Model file for the job. Use its own axes, mm. A direction names the side the tool comes from. Give positions to 0.01 mm unless a question says otherwise; leave off trailing zeros. Loops run counter-clockwise (first coordinate to the right, second up) from the corner with the lowest first, then second, coordinate; pieces in that order, holes last. Notation, with made-up numbers: (69.5, 3.5) - (82.5, 3.5) arc R35 cw to (82.5, 40.5) - close; hole circle Ø6 at (38, -6). An arc over 180 degrees is marked (long way). Use a Markdown table: item, result.
from build123d import *

# Parameters (mm, degrees)
SKETCH1_W               = 115
SKETCH1_H               = 55
SKETCH1_W_2             = 107
SKETCH1_H_2             = 47
BOSS_EXTRUDE1_DEPTH     = 6
SKETCH2_W               = 5
SKETCH2_H               = 2
BOSS_EXTRUDE2_DEPTH     = 8.5
CUT_EXTRUDE1_DEPTH      = 10
MIRROR2_COPY_1_SKETCH_W = 5
MIRROR2_COPY_1_SKETCH_H = 2
MIRROR2_COPY_1_DEPTH    = 8.5
MIRROR2_COPY_2_DEPTH    = 10
MIRROR3_COPY_1_SKETCH_W = 5
MIRROR3_COPY_1_SKETCH_H = 2
MIRROR3_COPY_1_DEPTH    = 8.5
MIRROR3_COPY_2_DEPTH    = 10
MIRROR3_COPY_3_SKETCH_W = 5
MIRROR3_COPY_3_SKETCH_H = 2
MIRROR3_COPY_3_DEPTH    = 8.5
MIRROR3_COPY_4_DEPTH    = 10
MIRROR3_COPY_5_SKETCH_W = 5
MIRROR3_COPY_5_SKETCH_H = 2
MIRROR3_COPY_5_DEPTH    = 8.5
MIRROR3_COPY_6_DEPTH    = 10


with BuildPart() as part:
    # Sketch1 → Boss-Extrude1 (new body)
    with BuildSketch(Plane.XY):
        Rectangle(SKETCH1_W, SKETCH1_H)
        Rectangle(SKETCH1_W_2, SKETCH1_H_2, mode=Mode.SUBTRACT)
    extrude(amount=BOSS_EXTRUDE1_DEPTH)

    # Sketch2 → Boss-Extrude2 (add)
    with BuildSketch(Plane.XY.offset(6)):
        with Locations((-42.5, 24.5)):
            Rectangle(SKETCH2_W, SKETCH2_H)
    boss_extrude2 = extrude(amount=BOSS_EXTRUDE2_DEPTH)

    # Sketch3 → Cut-Extrude1 (cut)
    with BuildSketch(Plane(origin=(-40, 0, 0), x_dir=(0, 0, -1), z_dir=(1, 0, 0))):
        Polygon((-14.5, 24.5), (-11, 25.5), (-11, 24.633842956), (-6, 24.633842956), (-6, 26.874562864), (-14.5, 26.874562864), align=None)
    cut_extrude1 = extrude(amount=-CUT_EXTRUDE1_DEPTH, mode=Mode.SUBTRACT)

    # Mirror1: Boss-Extrude2, Cut-Extrude1 across plane
    add(boss_extrude2.mirror(Plane.ZX))
    add(cut_extrude1.mirror(Plane.ZX), mode=Mode.SUBTRACT)

    # Mirror2: Boss-Extrude2, Cut-Extrude1 across plane
    add(boss_extrude2.mirror(Plane(origin=(0, 0, 0), x_dir=(0, 0, 1), z_dir=(1, 0, 0))))
    add(cut_extrude1.mirror(Plane(origin=(0, 0, 0), x_dir=(0, 0, 1), z_dir=(1, 0, 0))), mode=Mode.SUBTRACT)

    # Mirror2 copy 1 sketch → Mirror2 copy 1 (add)
    with BuildSketch(Plane(origin=(0, 0, 6), x_dir=(-1, 0, 0), z_dir=(0, 0, 1))):
        with Locations((-42.5, 24.5)):
            Rectangle(MIRROR2_COPY_1_SKETCH_W, MIRROR2_COPY_1_SKETCH_H)
    extrude(amount=MIRROR2_COPY_1_DEPTH)

    # Mirror2 copy 2 sketch → Mirror2 copy 2 (cut)
    with BuildSketch(Plane(origin=(40, 0, 0), x_dir=(0, 0, -1), z_dir=(-1, 0, 0))):
        Polygon((-14.5, 24.5), (-11, 25.5), (-11, 24.633842956), (-6, 24.633842956), (-6, 26.874562864), (-14.5, 26.874562864), align=None)
    extrude(amount=-MIRROR2_COPY_2_DEPTH, mode=Mode.SUBTRACT)

    # Mirror3: Boss-Extrude2, Cut-Extrude1 across plane
    add(boss_extrude2.mirror(Plane.XY.offset(3)))
    add(cut_extrude1.mirror(Plane.XY.offset(3)), mode=Mode.SUBTRACT)

    # Mirror3 copy 1 sketch → Mirror3 copy 1 (add)
    with BuildSketch(Plane(origin=(0, 0, 0), x_dir=(-1, 0, 0), z_dir=(0, 0, -1))):
        with Locations((-42.5, 24.5)):
            Rectangle(MIRROR3_COPY_1_SKETCH_W, MIRROR3_COPY_1_SKETCH_H)
    extrude(amount=MIRROR3_COPY_1_DEPTH)

    # Mirror3 copy 2 sketch → Mirror3 copy 2 (cut)
    with BuildSketch(Plane(origin=(40, 0, 6), x_dir=(0, 0, 1), z_dir=(-1, 0, 0))):
        Polygon((-14.5, 24.5), (-11, 25.5), (-11, 24.633842956), (-6, 24.633842956), (-6, 26.874562864), (-14.5, 26.874562864), align=None)
    extrude(amount=-MIRROR3_COPY_2_DEPTH, mode=Mode.SUBTRACT)

    # Mirror3 copy 3 sketch → Mirror3 copy 3 (add)
    with BuildSketch(Plane(origin=(0, 0, 0), x_dir=(-1, 0, 0), z_dir=(0, 0, -1))):
        with Locations((-42.5, -24.5)):
            Rectangle(MIRROR3_COPY_3_SKETCH_W, MIRROR3_COPY_3_SKETCH_H)
    extrude(amount=MIRROR3_COPY_3_DEPTH)

    # Mirror3 copy 4 sketch → Mirror3 copy 4 (cut)
    with BuildSketch(Plane(origin=(40, 0, 6), x_dir=(0, 0, 1), z_dir=(-1, 0, 0))):
        Polygon((-14.5, -24.5), (-11, -25.5), (-11, -24.633842956), (-6, -24.633842956), (-6, -26.874562864), (-14.5, -26.874562864), align=None)
    extrude(amount=-MIRROR3_COPY_4_DEPTH, mode=Mode.SUBTRACT)

    # Mirror3 copy 5 sketch → Mirror3 copy 5 (add)
    with BuildSketch(Plane(origin=(0, 0, 0), x_dir=(1, 0, 0), z_dir=(0, 0, -1))):
        with Locations((-42.5, 24.5)):
            Rectangle(MIRROR3_COPY_5_SKETCH_W, MIRROR3_COPY_5_SKETCH_H)
    extrude(amount=MIRROR3_COPY_5_DEPTH)

    # Mirror3 copy 6 sketch → Mirror3 copy 6 (cut)
    with BuildSketch(Plane(origin=(-40, 0, 6), x_dir=(0, 0, 1), z_dir=(1, 0, 0))):
        Polygon((-14.5, 24.5), (-11, 25.5), (-11, 24.633842956), (-6, 24.633842956), (-6, 26.874562864), (-14.5, 26.874562864), align=None)
    extrude(amount=-MIRROR3_COPY_6_DEPTH, mode=Mode.SUBTRACT)


solid = part.part
(1) 3-axis set-ups, long thin cutter, end or side, ignore diameter. For faces 1 (the flat face through (-40, -24, -4)), 2 (the flat face through (45, -24, -4)), 3 (the flat face through (42, -24.634, 9)), 4 (the flat face through (-42, 24.634, -3)): which of +Z, -Z, +X, -X, +Y, -Y reach the whole face in a straight line?
Computed:
| item | result |
|---|---|
| face 1 | -Z, +Y, -Y |
| face 2 | -Z, +X, +Y, -Y |
| face 3 | +X, -X, -Y |
| face 4 | +X, -X, +Y |
(2) Slice it at C-C, the plane x = 27. Write the cut outline in (y, z), plus the area to 3 significant figures.
Computed:
| item | result |
|---|---|
| outline | (-27.5, 0) - (-23.5, 0) - (-23.5, 6) - (-27.5, 6) - close; (23.5, 0) - (27.5, 0) - (27.5, 6) - (23.5, 6) - close |
| area | 48.0 mm² |
(3) Slice it at B-B, the plane z = 8. Write the cut outline in (x, y), plus the area to 3 significant figures.
Computed:
| item | result |
|---|---|
| outline | (-45, -24.63) - (-40, -24.63) - (-40, -23.5) - (-45, -23.5) - close; (-45, 23.5) - (-40, 23.5) - (-40, 24.63) - (-45, 24.63) - close; (40, -24.63) - (45, -24.63) - (45, -23.5) - (40, -23.5) - close; (40, 23.5) - (45, 23.5) - (45, 24.63) - (40, 24.63) - close |
| area | 22.7 mm² |
(4) Mould opens along Z. For faces 5 (the flat face through (53.5, 0, 3)), 6 (the flat face through (42.465, 24.993, -6.774)), 7 (the flat face through (-42, 24.634, 9)) say: pulls with the +Z half, pulls with the -Z half, needs draft (parallel to the pull), parting line crosses it, or undercut.
Computed:
| item | result |
|---|---|
| face 5 | needs draft |
| face 6 | pulls with the -Z half |
| face 7 | undercut |
(5) Drill centre lines: probe 1 along Y at (x, z) = (-37, 1.75); probe 2 along X at (y, z) = (19, 4.5); probe 3 along X at (y, z) = (24, 9.75). Where is each one in solid material? Low to high. Write a range as [from, to].
Computed:
| item | result |
|---|---|
| probe 1 | [-27.5, -23.5], [23.5, 27.5] |
| probe 2 | [-57.5, -53.5], [53.5, 57.5] |
| probe 3 | [-45, -40], [40, 45] |
(6) Slice it at A-A, the plane y = 21.5. Write the cut outline in (x, z).
Computed:
| item | result |
|---|---|
| outline | (-57.5, 0) - (-53.5, 0) - (-53.5, 6) - (-57.5, 6) - close; (53.5, 0) - (57.5, 0) - (57.5, 6) - (53.5, 6) - close |
(7) Slice it at D-D, the plane z = 12.75. Write the cut outline in (x, y), plus the area to 3 significant figures.
Computed:
| item | result |
|---|---|
| outline | (-45, -25) - (-40, -25) - (-40, -23.5) - (-45, -23.5) - close; (-45, 23.5) - (-40, 23.5) - (-40, 25) - (-45, 25) - close; (40, -25) - (45, -25) - (45, -23.5) - (40, -23.5) - close; (40, 23.5) - (45, 23.5) - (45, 25) - (40, 25) - close |
| area | 30.0 mm² |
(8) Pin check, flat tips, straight feed: P1, Ø2, axis at y = 25, z = -4.5, coming from the -X side; P2, Ø2.5, axis at x = 43.5, z = 9, coming from the -Y side; P3, Ø1.5, axis at x = 42.5, z = -3, coming from the +Y side; P4, Ø10, axis at y = -10.5, z = 11.5, coming from the -X side. Stop position of each tip, or through.
Computed:
| item | result |
|---|---|
| P1 | x = -45 |
| P2 | y = -24.63 |
| P3 | y = 24.63 |
| P4 | through |
